from build123d import *

# Parameters (mm, degrees)
SKETCH2_R           = 2.2
BOSS_EXTRUDE1_DEPTH = 12.7


with BuildPart() as part:
    # Sketch2 → Boss-Extrude1 (new body)
    with BuildSketch(Plane(origin=(0, 0, 0), x_dir=(0, 0, -1), z_dir=(1, 0, 0))):
        with BuildLine():
            Line((-75, 155), (45, 155))
            ThreePointArc((45, 155), (50, 150), (45, 145))
            Line((45, 145), (-72.928932188, 145))
            Line((-72.928932188, 145), (-113.890872965, 104.038059223))
            ThreePointArc((-113.890872965, 104.038059223), (-120.961940777, 104.038059223), (-120.961940777, 111.109127035))
            Line((-120.961940777, 111.109127035), (-78.535533906, 153.535533906))
            ThreePointArc((-78.535533906, 153.535533906), (-76.913417162, 154.619397663), (-75, 155))
        make_face()
        with Locations((-5, 150)):
            Circle(SKETCH2_R, mode=Mode.SUBTRACT)
        with Locations((45, 150)):
            Circle(SKETCH2_R, mode=Mode.SUBTRACT)
    extrude(amount=BOSS_EXTRUDE1_DEPTH)


solid = part.part
Design review of the part built by this model. Coordinates are the model's own, in mm. Coordinates: 2 decimals unless noted, no trailing zeros. Loops run counter-clockwise (first coordinate to the right, second up) from the corner with the lowest first, then second, coordinate; pieces in that order, holes last. Notation, with made-up numbers: M -13.75,59 L 34.25,59 A9 cw 34.25,65 Z; hole C 76,22 d7. An arc over 180 degrees is marked long. Use one line per item in the form item = value.
(1) Consider section D-D (y = 122.5). Write out the cut boundary in (x, z), and give its area (3 significant figures).
Return value:
outline = M 0,95.43 L 12.7,95.43 L 12.7,109.57 L 0,109.57 Z
area = 180 mm2
(2) Consider section C-C (z = -7.5). Write out the cut boundary in (x, y), and give its area (3 significant figures).
Return value:
outline = M 0,145 L 12.7,145 L 12.7,155 L 0,155 Z
area = 127 mm2
(3) Clearance check with flat-ended pins moving along their axes: P1, Ø1, axis at x = 3.5, y = 113.5, coming from the -Z side; P2, Ø3, axis at x = 5.5, z = 101.5, coming from the +Y side; P3, Ø2, axis at x = 7, y = 128.5, coming from the -Z side. State where each tip first meets the part, or that it passes through.
Return value:
P1 = 103.93
P2 = 132.07
P3 = 88.43
(4) Consider section A-A (x = 3.25). Write out the cut boundary in (y, z).
Return value:
outline = M 104.04,113.89 L 145,72.93 L 145,-45 A5 ccw 155,-45 L 155,75 A5 ccw 153.54,78.54 L 111.11,120.96 A5 ccw Z; hole C 150,-45 d4.4; hole C 150,5 d4.4
(5) Draft analysis for pull direction Y (two halves, no side actions). For faces 1 (the face through (6, 145, 13)), 2 (the face through (12.7, 148, 42)), 3 (the face through (6.261, 151.855, 3.817)), 4 (the face through (6.26, 151.49, -43.38)), state which applies: pulls with the +Y half, pulls with the -Y half, needs draft (parallel to the pull), parting line crosses it, or undercut.
Return value:
face_1 = pulls with the -Y half
face_2 = needs draft
face_3 = undercut
face_4 = undercut
(6) Consider section B-B (y = 150). Write out the cut boundary in (x, z), and give its area (3 significant figures).
Return value:
outline = M 0,-50 L 12.7,-50 L 12.7,-47.2 L 0,-47.2 Z; M 0,-42.8 L 12.7,-42.8 L 12.7,2.8 L 0,2.8 Z; M 0,7.2 L 12.7,7.2 L 12.7,82.07 L 0,82.07 Z
area = 1,570 mm2
(7) For line 1 along Z through (x, y) = (3.25, 150); line 2 along Y through (x, z) = (7, -45); line 3 along Y through (x, z) = (8.5, 19), list the stretches that pass through material, from the lowest coordinate up. Write a range as from..to.
Return value:
line_1 = -50..-47.2, -42.8..2.8, 7.2..82.07
line_2 = 145..147.8, 152.2..155
line_3 = 145..155
